```python
from build123d import *

# Parameters (mm, degrees)
SKETCH1_W                                            = 190.5
SKETCH1_H                                            = 76.2
EXTRUDE1_DEPTH                                       = 12.7
SIDE_1_4_20_TAPPED_HOLE_MASTER_AT_2_COUNT            = 2
SIDE_1_4_20_TAPPED_HOLE_MASTER_AT_2_PITCH            = 46.228697797
TOP_1_4_20_TAPPED_HOES_D                             = 5.1054
BUSIHING_FLEXURE_COUPLING_1_4_20_BOLT_HO_D           = 6.7564
BUSIHING_FLEXURE_COUPLING_1_4_20_BOLT_HO_CBORE_D     = 11.1125
BUSIHING_FLEXURE_COUPLING_1_4_20_BOLT_HO_CBORE_DEPTH = 6.35
LEAD_SCREW_1_4_CAP_SCREW_MOUNTS_D                    = 6.7564
LEAD_SCREW_1_4_CAP_SCREW_MOUNTS_CBORE_D              = 11.1125
LEAD_SCREW_1_4_CAP_SCREW_MOUNTS_CBORE_DEPTH          = 6.35


with BuildPart() as part:
    # Sketch1 → Extrude1 (new, symmetric)
    with BuildSketch(Plane.XY):
        Rectangle(SKETCH1_W, SKETCH1_H)
    extrude(amount=EXTRUDE1_DEPTH, both=True)

    # Sketch10 → Side-1/4-20 tapped hole master (revolve, cut)
    with BuildSketch(Plane(origin=(22.225, -38.1, 6.35), x_dir=(0, 0, -1), z_dir=(1, 0, 0))):
        Polygon((0, 0), (0, 20.583816902), (2.5527, 19.05), (2.5527, 0), align=None)
    side_1_4_20_tapped_hole_master = revolve(axis=Axis((22.225, -44.45, 6.35), (0, 1, 0)), mode=Mode.SUBTRACT)

    # Side-1/4-20 tapped hole master at 2: Side-1/4-20 tapped hole master ×2
    with Locations(*[Vector(0.9615239476408232, 0, -0.27472112789737807) * (i * SIDE_1_4_20_TAPPED_HOLE_MASTER_AT_2_PITCH) for i in range(1, SIDE_1_4_20_TAPPED_HOLE_MASTER_AT_2_COUNT)]):
        add(side_1_4_20_tapped_hole_master, mode=Mode.SUBTRACT)

    # Side-1/4-20 tapped hole mirror I: Side-1/4-20 tapped hole master across plane
    add(side_1_4_20_tapped_hole_master.mirror(Plane(origin=(0, 0, 0), x_dir=(0, 0, 1), z_dir=(1, 0, 0))), mode=Mode.SUBTRACT)

    # Side-1/4-20 tapped hole mirror I copy 1 → Side-1/4-20 tapped hole mirror I cop 2 (revolve, cut)
    with BuildSketch(Plane(origin=(-66.675, -38.1, -6.35), x_dir=(0, 0, -1), z_dir=(-1, 0, 0))):
        Polygon((0, 0), (0, -20.583816902), (2.5527, -19.05), (2.5527, 0), align=None)
    revolve(axis=Axis((-66.675, -44.45, -6.35), (0, -1, 0)), mode=Mode.SUBTRACT)

    # Side-1/4-20 tapped hole mirror II: Side-1/4-20 tapped hole master across plane
    add(side_1_4_20_tapped_hole_master.mirror(Plane.ZX), mode=Mode.SUBTRACT)

    # Side-1/4-20 tapped hole mirror II copy 1 → Side-1/4-20 tapped hole mirror II co 2 (revolve, cut)
    with BuildSketch(Plane(origin=(66.675, 38.1, -6.35), x_dir=(0, 0, -1), z_dir=(1, 0, 0))):
        Polygon((0, 0), (0, -20.583816902), (2.5527, -19.05), (2.5527, 0), align=None)
    revolve(axis=Axis((66.675, 44.45, -6.35), (0, 1, 0)), mode=Mode.SUBTRACT)

    # Side-1/4-20 tapped hole mirror II copy 2 → Side-1/4-20 tapped hole mirror II co 3 (revolve, cut)
    with BuildSketch(Plane(origin=(-22.225, 38.1, 6.35), x_dir=(0, 0, -1), z_dir=(-1, 0, 0))):
        Polygon((0, 0), (0, 20.583816902), (2.5527, 19.05), (2.5527, 0), align=None)
    revolve(axis=Axis((-22.225, 44.45, 6.35), (0, -1, 0)), mode=Mode.SUBTRACT)

    # Side-1/4-20 tapped hole mirror II copy 3 → Side-1/4-20 tapped hole mirror II co 4 (revolve, cut)
    with BuildSketch(Plane(origin=(-66.675, 38.1, -6.35), x_dir=(0, 0, -1), z_dir=(-1, 0, 0))):
        Polygon((0, 0), (0, 20.583816902), (2.5527, 19.05), (2.5527, 0), align=None)
    revolve(axis=Axis((-66.675, 44.45, -6.35), (0, -1, 0)), mode=Mode.SUBTRACT)

    # Top-1/4-20 tapped hoes (through all)
    with Locations(Plane.XY.offset(12.7)):
        with Locations((-61.849, 19.05), (-61.849, -19.05), (-87.249, 19.05), (-87.249, -19.05), (87.249, 19.05), (87.249, -19.05), (61.849, 19.05), (61.849, -19.05)):
            Hole(TOP_1_4_20_TAPPED_HOES_D / 2)

    # Busihing flexure coupling 1/4-20 bolt holes (through all)
    with Locations(Plane(origin=(-12.155752838, -9.35929282, 12.7), x_dir=(-1, 0, 0), z_dir=(0, 0, 1))):
        with Locations((-56.605752838, -9.35929282), (-82.005752838, -9.35929282)):
            CounterBoreHole(BUSIHING_FLEXURE_COUPLING_1_4_20_BOLT_HO_D / 2, BUSIHING_FLEXURE_COUPLING_1_4_20_BOLT_HO_CBORE_D / 2, BUSIHING_FLEXURE_COUPLING_1_4_20_BOLT_HO_CBORE_DEPTH)

    # Lead screw 1/4 cap screw mounts (through all)
    with Locations(Plane(origin=(36.480699887, 13.8528382, 12.7), x_dir=(-1, 0, 0), z_dir=(0, 0, 1))):
        with Locations((36.480699887, 5.9153382), (36.480699887, 21.7903382)):
            CounterBoreHole(LEAD_SCREW_1_4_CAP_SCREW_MOUNTS_D / 2, LEAD_SCREW_1_4_CAP_SCREW_MOUNTS_CBORE_D / 2, LEAD_SCREW_1_4_CAP_SCREW_MOUNTS_CBORE_DEPTH)


solid = part.part
```
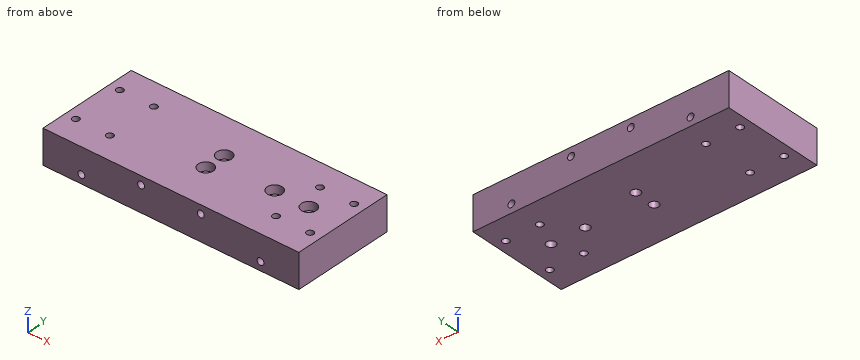
Geometry check sheet. Reference: the model listing, model coordinates, mm. Round coordinates to 2 decimals unless told otherwise and drop trailing zeros. Order: outer loops, then holes, each group sorted by start corner. A loop starts at its lowest first (then second) coordinate and runs counter-clockwise, first axis right, second up. Notation, with made-up numbers: M 10,75.5 L 66,75.5 A19 cw 66,110.5 Z; hole C 10,-14 d4. An arc over 180 degrees is marked long. Answer as CSV lines item,"result".
1) Sectioned sample at C-C on z = 10.75. Give the number of separate pieces and of enclosed holes in the cut face, and give its area (3 significant figures).
Entries:
separate pieces,"1"
enclosed holes,"12"
area,"14,000 mm2"
2) Thickness scan on probe 1 along X at (y, z) = (-19.5, -10); probe 2 along Y at (x, z) = (62, -5.25); probe 3 along X at (y, z) = (-30, 7). Record the ranges inside material, lowest first. Write a range as [from, to].
Entries:
probe 1,"[-95.25, -89.76], [-84.74, -64.36], [-59.34, 59.34], [64.36, 84.74], [89.76, 95.25]"
probe 2,"[-38.1, -21.6], [-16.5, 16.5], [21.6, 38.1]"
probe 3,"[-95.25, -24.69], [-19.76, 19.76], [24.69, 95.25]"
3) Gauge pin test, flat end, axial feed: pin 1 Ø5.5 at (x, y) = (70.5, -2) entering from +Z. Record the tip position at first contact, or that the pin passes through.
Entries:
pin 1,"z = 6.35"
4) Sectioned sample at A-A on x = 44.45. Record the cut outline in (y, z).
Entries:
outline,"M -38.1,-12.7 L -3.38,-12.7 L -3.38,6.35 L -5.56,6.35 L -5.56,12.7 L -38.1,12.7 Z; M 3.38,-12.7 L 38.1,-12.7 L 38.1,12.7 L 5.56,12.7 L 5.56,6.35 L 3.38,6.35 Z"
5) Sectioned sample at B-B on y = 0. Record the cut outline in (x, z).
Entries:
outline,"M -95.25,-12.7 L 41.07,-12.7 L 41.07,6.35 L 38.89,6.35 L 38.89,12.7 L -95.25,12.7 Z; M 47.83,-12.7 L 66.47,-12.7 L 66.47,6.35 L 64.29,6.35 L 64.29,12.7 L 50.01,12.7 L 50.01,6.35 L 47.83,6.35 Z; M 73.23,-12.7 L 95.25,-12.7 L 95.25,12.7 L 75.41,12.7 L 75.41,6.35 L 73.23,6.35 Z"
6) Sectioned sample at D-D on y = 26. Record the cut outline in (x, z) (3 decimals), and give its area (3 significant figures).
Entries:
outline,"M -95.25,-12.7 L 95.25,-12.7 L 95.25,12.7 L -95.25,12.7 Z; hole C -66.675,-6.35 d5.105; hole C -22.225,6.35 d5.105; hole C 22.225,6.35 d5.105; hole C 66.675,-6.35 d5.105"
area,"4,760 mm2"
